Check sheet for the drawn part. Datum: minimum x, y, z corner. Units: mm. A direction names the side the tool comes from. Coordinates: 2 decimals unless noted, no trailing zeros. Loops run counter-clockwise (first coordinate to the right, second up) from the corner with the lowest first, then second, coordinate; pieces in that order, holes last.
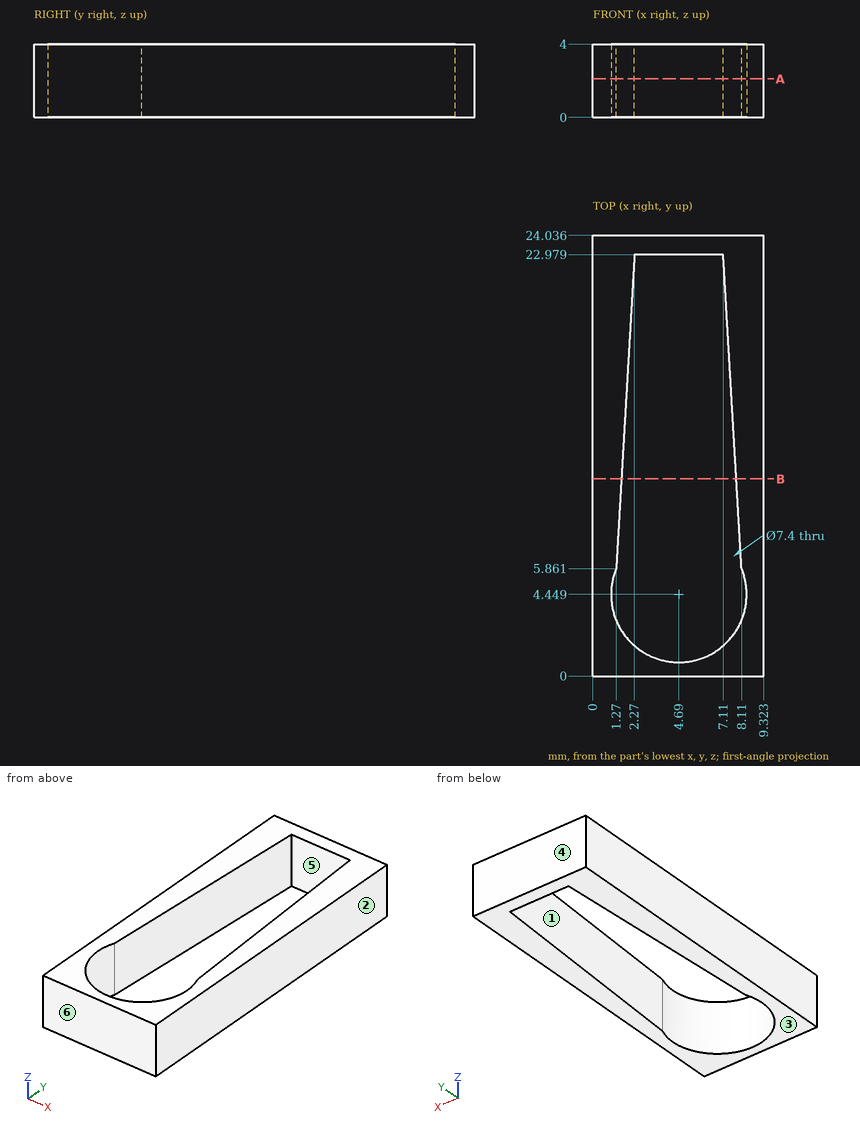
1) Mould release check, pull along Y, two halves, no side actions. Record for the marked faces 3, 4, 5 and 6: +Y half, -Y half, draft (parallel to the pull), parting line (faces both ways), or undercut.
Answer sheet:
face 3: draft
face 4: +Y half
face 5: undercut
face 6: -Y half
2) Section check A-A on z = 2.1. Enter the section's corners in (x, y) (1 decimal).
Answer sheet:
outline: (0, 0) - (9.3, 0) - (9.3, 24) - (0, 24) - close; hole (1.3, 5.9) arc R3.7 ccw (long way) to (8.1, 5.9) - (7.1, 23) - (2.3, 23) - close
3) Scan lines: line 1 (X direction, y = 4.5, z = 0.3); line 2 (Y direction, x = 6, z = 1) (1 decimal); line 3 (X direction, y = 10.5, z = 2.4). Record each from-to range of solid material in increasing order.
Answer sheet:
line 1: x = 0 to 0.99, 8.39 to 9.32
line 2: y = 0 to 1, 23 to 24
line 3: x = 0 to 1.54, 7.84 to 9.32
4) Set-up check for the marked faces 1 and 2: record each of +Z, -Z, +X, -X, +Y, -Y from which the full face is reachable in a straight line by a thin tool's end or side.
Answer sheet:
face 1: +Z, -Z
face 2: +Z, -Z, +X, +Y, -Y
5) Section check B-B on y = 10.75. Enter the section's corners in (x, z) (1 decimal).
Answer sheet:
outline: (0, 0) - (1.6, 0) - (1.6, 4) - (0, 4) - close; (7.8, 0) - (9.3, 0) - (9.3, 4) - (7.8, 4) - close
